Autodesk Inventor part; units mm, degrees
ref_plane "YZ Plane" through (0, 0, 0) normal (1, 0, 0) x (0, 1, 0)
ref_plane "XZ Plane" through (0, 0, 0) normal (0, 1, 0) x (-1, 0, 0)
ref_plane "XY Plane" through (0, 0, 0) normal (0, 0, 1) x (1, 0, 0)
sketch "Sketch1" plane through (0, 0, 0) normal (0, 0, 1) x (1, 0, 0)
  line L0 (142.5, 18) -> (-142.5, 18)
  line L1 (-142.5, 18) -> (-142.5, -18)
  line L2 (-142.5, -18) -> (142.5, -18)
  line L3 (142.5, -18) -> (142.5, 18)
  line L4 (142.5, 18) -> (-142.5, -18) construction
  line L5 (-142.5, 18) -> (142.5, -18) construction
  line L6 (-142.5, 18) -> (142.5, 18)
  line L7 (142.5, 18) -> (142.5, 8)
  line L8 (142.5, 8) -> (-142.5, 8)
  line L9 (-142.5, 8) -> (-142.5, 18)
  point P0 (0, 0)
  point P1 (142.5, 13)
  dimension "d0" = 285
  dimension "d1" = 36
  dimension "d4" = 5
extrude "Extrusion1" add sketch "Sketch1" along normal blind 10
sketch "Sketch4" plane through (0, 0, 10) normal (0, 0, 1) x (1, 0, 0)
  line L0 (-142.5, 18) -> (-142.5, -18)
  line L1 (-142.5, 18) -> (142.5, 18)
  line L2 (142.5, 18) -> (142.5, 13)
  line L3 (142.5, 13) -> (-142.5, 13)
  line L4 (-142.5, 13) -> (-142.5, 18)
  point P0 (0, 0)
  dimension "d5" = 285
  dimension "d6" = 5
extrude "Extrusion2" add sketch "Sketch4" along normal blind 15
sketch "Sketch5" plane through (0, 0, 10) normal (0, 0, 1) x (1, 0, 0)
  line L0 (-142.5, 18) -> (-142.5, -18)
  line L1 (-142.5, 7) -> (142.5, 7)
  line L2 (142.5, 7) -> (142.5, 2)
  line L3 (142.5, 2) -> (-142.5, 2)
  line L4 (-142.5, 2) -> (-142.5, 7)
  line L5 (142.5, 13) -> (-142.5, 13)
  point P0 (0, 0)
  dimension "d9" = 285
  dimension "d10" = 5
  dimension "d47" = 11
extrude "Extrusion3" add sketch "Sketch5" along normal blind 15
fillet "Fillet1" radius 7.5 1 edges at (0, 2, 10)
sketch "Sketch6" plane through (0, 0, 10) normal (0, 0, 1) x (1, 0, 0)
  circle A0 centre (-70, -8.5) radius 2.5
  line L0 (-142.5, -5.5) -> (142.5, -5.5)
  line L1 (-142.5, -18) -> (142.5, -18)
  point P0 (0, 0)
  point P1 (0, -5.5)
  point P2 (0, -5.5)
  dimension "d50" = 70
  dimension "d51" = 9.5
hole "Hole1" at (-70, -8.5, 10) direction (0, 0, -1) diameter 5 end through all
sketch "Sketch7" plane through (0, 0, 10) normal (0, 0, 1) x (1, 0, 0)
  circle A0 centre (0, -8.5) radius 2.5
  circle A1 centre (-70, -8.5) radius 2.5
  line L0 (-142.5, -18) -> (142.5, -18)
  point P0 (0, 0)
  point P1 (-69.25, -4.8686)
  point P2 (-64.25, -4.8686)
  dimension "d23" = 5
  dimension "d39" = 70
  dimension "d43" = 9.5
hole "Hole2" at (0, -8.5, 10) direction (0, 0, -1) diameter 5 end through all
sketch "Sketch8" plane through (0, 0, 10) normal (0, 0, 1) x (1, 0, 0)
  circle A0 centre (69.4481, -8.5) radius 2.5
  circle A1 centre (0, -8.5) radius 2.5
  line L0 (-142.5, -5.5) -> (142.5, -5.5)
  line L1 (-142.5, -18) -> (142.5, -18)
  point P0 (0, 0)
  point P1 (-1.3066, -5.3686)
  point P2 (1.3066, -5.3686)
  point P3 (-70, -4.8686)
  dimension "d31" = 5
  dimension "d48" = 7
hole "Hole3" at (69.4481, -8.5, 10) direction (0, 0, -1) diameter 5 end through all
properties part number "side part v3"
The model under review builds one solid part; all positions refer to its coordinate system, in mm. A direction names the side the tool comes from. Give positions to 0.01 mm unless a question says otherwise; leave off trailing zeros. Write each loop counter-clockwise with the first axis right and the second up, starting at its lowest first coordinate (ties: lowest second). Pieces come first, ordered by that corner, then holes.
(1) Consider section B-B, the plane x = 0. Give the boundary of the cut face in (y, z).
(2) For P1, Ø2, axis at x = 48.5, y = 5.5, coming from the -Z side; P2, Ø5, axis at x = 49, z = 19, coming from the -Y side; P3, Ø4.5, axis at x = 5, z = 20.5, coming from the -Y side; P4, Ø5, axis at x = 67.5, y = -2, coming from the +Z side, all flat-tipped, find the tip position at first contact; note any pin that passes through.
(3) Consider section D-D, the plane y = 9.5. Give the boundary of the cut face in (x, z), and give its area (3 significant figures).
(4) The part is to be moulded in two halves that separate along X. For faces 1 (the flat face through (-2, 18, 12)), 2 (the cylindrical face through (67, -8, 5)), 3 (the flat face through (142.5, 4, 10)), say which applies: released by +X, released by -X, zero draft, split by the parting line, or undercut.
(5) To check wall thickness, follow L1, parallel to X at y = -8.5, z = 3; L2, parallel to Y at x = -70, z = 4.75; L3, parallel to Y at x = 126, z = 19.25. State the ranges of each line that lie inside material, in increasing order.
(6) Tool access review of faces 4 (the flat face through (-2, 0, 0)), 5 (the flat face through (2, 2, 21)), 6 (the flat face through (-2, 10, 10)): name each direction out of +Z, -Z, +X, -X, +Y, -Y from which nothing blocks a thin tool from reaching the whole face with its end or side.
(7) Consider section A-A, the plane y = -8.5. Give the boundary of the cut face in (x, z).
(8) Consider section C-C, the plane x = -32. Give the boundary of the cut face in (y, z).
Returned:
1. outline: (-18, 0) - (-11, 0) - (-11, 10) - (-18, 10) - close; (-6, 0) - (18, 0) - (18, 25) - (13, 25) - (13, 10) - (7, 10) - (7, 25) - (2, 25) - (2, 17.5) arc R7.5 cw to (-5.5, 10) - (-6, 10) - close
2. P1: stops at z = 0
2. P2: stops at y = 1.93
2. P3: stops at y = 2
2. P4: stops at z = 13
3. outline: (-142.5, 0) - (142.5, 0) - (142.5, 10) - (-142.5, 10) - close
3. area: 2,850 mm2
4. face 1: zero draft
4. face 2: undercut
4. face 3: released by +X
5. L1: x = -142.5 to -72.5, -67.5 to -2.5, 2.5 to 66.95, 71.95 to 142.5
5. L2: y = -18 to -11, -6 to 18
5. L3: y = 2 to 7, 13 to 18
6. face 4: -Z, +X, -X, +Y, -Y
6. face 5: +Z, +X, -X, -Y
6. face 6: +Z, +X, -X
7. outline: (-142.5, 0) - (-72.5, 0) - (-72.5, 10) - (-142.5, 10) - close; (-67.5, 0) - (-2.5, 0) - (-2.5, 10) - (-67.5, 10) - close; (2.5, 0) - (66.95, 0) - (66.95, 10) - (2.5, 10) - close; (71.95, 0) - (142.5, 0) - (142.5, 10) - (71.95, 10) - close
8. outline: (-18, 0) - (18, 0) - (18, 25) - (13, 25) - (13, 10) - (7, 10) - (7, 25) - (2, 25) - (2, 17.5) arc R7.5 cw to (-5.5, 10) - (-18, 10) - close
